Here's how the part is built. I have some questions about the finished solid (model axes, mm). Face numbers are marked on the shaded views. A direction names the side the tool comes from. Coordinates: 2 decimals unless noted, no trailing zeros. Loops run counter-clockwise (first coordinate to the right, second up) from the corner with the lowest first, then second, coordinate; pieces in that order, holes last. Notation, with made-up numbers: (-36, 28.5) - (-27, 28.5) arc R8 ccw to (-27, 34.5) - close; hole circle Ø2 at (26.5, 4.5). An arc over 180 degrees is marked (long way). Use a Markdown table: item, result.
```python
from build123d import *

# Parameters (mm, degrees)
BOSS_EXTRUDE1_DEPTH = 118.4275
SKETCH3_R           = 3.96875
SKETCH3_R_2         = 6.5
CUT_EXTRUDE1_DEPTH  = 25.4
SKETCH6_R           = 3.96875
CUT_EXTRUDE3_DEPTH  = 8.89
SKETCH4_R           = 4.7625
CUT_EXTRUDE2_DEPTH  = 6.35
SKETCH7_R           = 6.35
CUT_EXTRUDE4_DEPTH  = 2.54


with BuildPart() as part:
    # Sketch2 → Boss-Extrude1 (new body)
    with BuildSketch(Plane(origin=(0, 0, 0), x_dir=(0, 0, -1), z_dir=(1, 0, 0))):
        Polygon((0, -25.4), (0, 25.4), (-63.5, 25.4), (-63.5, 16.51), (-6.35, 16.51), (-6.35, -16.51), (-63.5, -16.51), (-63.5, -25.4), align=None)
    extrude(amount=BOSS_EXTRUDE1_DEPTH)

    # Sketch3 → Cut-Extrude1 (cut)
    with BuildSketch(Plane(origin=(0, 0, 0), x_dir=(1, 0, 0), z_dir=(0, 1, 0))):
        with Locations(Location((7.9375, -19.05, 0), (0, 0, 90))):
            Circle(SKETCH3_R)
        with Locations(Location((110.49, -19.05, 0), (0, 0, 90))):
            Circle(SKETCH3_R)
        with Locations(Location((38.1, -20.32, 0), (0, 0, 90))):
            Circle(SKETCH3_R_2)
        with BuildLine():
            Line((0, -63.5), (0, -19.05))
            ThreePointArc((0, -19.05), (1.173211717, -23.203108508), (4.346030936, -26.128506637))
            Line((4.346030936, -26.128506637), (30.73922523, -39.519797436))
            ThreePointArc((30.73922523, -39.519797436), (40.148824549, -41.564990827), (49.356556182, -38.747003333))
            Line((49.356556182, -38.747003333), (91.51717293, -12.752709815))
            ThreePointArc((91.51717293, -12.752709815), (93.758058641, -11.767067469), (96.182815356, -11.43))
            Line((96.182815356, -11.43), (98.7425, -11.43))
            ThreePointArc((98.7425, -11.43), (101.436576836, -12.545923164), (102.5525, -15.24))
            Line((102.5525, -15.24), (102.5525, -19.05))
            ThreePointArc((102.5525, -19.05), (110.49, -26.9875), (118.4275, -19.05))
            Line((118.4275, -19.05), (118.4275, -63.5))
            Line((118.4275, -63.5), (0, -63.5))
        make_face()
    extrude(amount=CUT_EXTRUDE1_DEPTH, mode=Mode.SUBTRACT)

    # Sketch6 → Cut-Extrude3 (cut)
    with BuildSketch(Plane.XZ.offset(25.4)):
        with Locations(Location((110.49, 19.05, 0), (0, 0, 270))):
            Circle(SKETCH6_R)
        with Locations(Location((7.9375, 19.05, 0), (0, 0, 270))):
            Circle(SKETCH6_R)
        with BuildLine():
            Line((0, 19.05), (0, 63.5))
            Line((0, 63.5), (118.4275, 63.5))
            Line((118.4275, 63.5), (118.4275, 19.05))
            ThreePointArc((118.4275, 19.05), (110.49, 26.9875), (102.5525, 19.05))
            Line((102.5525, 19.05), (102.5525, 15.24))
            ThreePointArc((102.5525, 15.24), (101.436576836, 12.545923164), (98.7425, 11.43))
            Line((98.7425, 11.43), (96.182815356, 11.43))
            ThreePointArc((96.182815356, 11.43), (93.758058641, 11.767067469), (91.51717293, 12.752709815))
            Line((91.51717293, 12.752709815), (60.419932998, 31.92583499))
            Line((60.419932998, 31.92583499), (15.772114941, 31.92583499))
            Line((15.772114941, 31.92583499), (4.346030936, 26.128506637))
            ThreePointArc((4.346030936, 26.128506637), (1.173211717, 23.203108508), (0, 19.05))
        make_face()
        with BuildLine():
            Line((25.6667, 27.370915615), (25.6667, 23.429084385))
            ThreePointArc((25.6667, 23.429084385), (20.0025, 25.4), (25.6667, 27.370915615))
        make_face()
    extrude(amount=-CUT_EXTRUDE3_DEPTH, mode=Mode.SUBTRACT)

    # Sketch4 → Cut-Extrude2 (cut)
    with BuildSketch(Plane.XY):
        with Locations(Location((19.05, 0, 0), (0, 0, 180))):
            Circle(SKETCH4_R)
        with Locations(Location((99.3775, 0, 0), (0, 0, 180))):
            Circle(SKETCH4_R)
    extrude(amount=CUT_EXTRUDE2_DEPTH, mode=Mode.SUBTRACT)

    # Sketch7 → Cut-Extrude4 (cut)
    with BuildSketch(Plane(origin=(0, -16.51, 0), x_dir=(1, 0, 0), z_dir=(0, 1, 0))):
        with Locations(Location((23.1775, -25.4, 0), (0, 0, 270))):
            Circle(SKETCH7_R)
    extrude(amount=-CUT_EXTRUDE4_DEPTH, mode=Mode.SUBTRACT)


solid = part.part
```
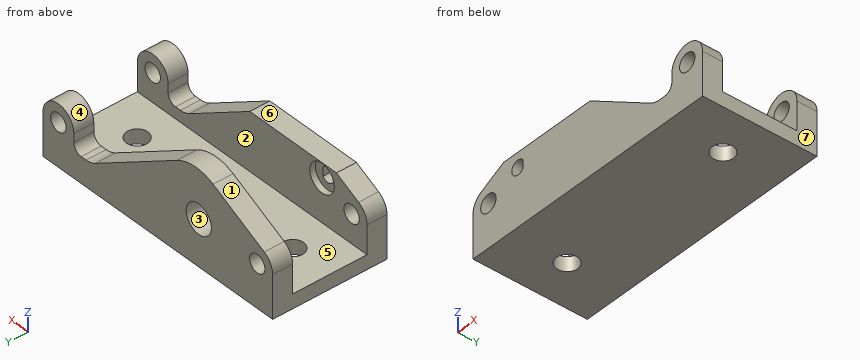
Q1. If we mould it in two halves opening along X, with no side actions, what happens to the marked faces 1, 2, 3 and 4? For each: pulls with the +X half, pulls with the -X half, needs draft (parallel to the pull), parting line crosses it, or undercut.
Check values:
| item | result |
|---|---|
| face 1 | pulls with the -X half |
| face 2 | needs draft |
| face 3 | undercut |
| face 4 | undercut |
Q2. Which directions (+Z, -Z, +X, -X, +Y, -Y) give clear straight access to the entire face, cutting with the end or side of a thin tool? Please do the marked faces 5, 6 and 7.
Check values:
| item | result |
|---|---|
| face 5 | +Z, +X, -X |
| face 6 | +Z, +X, -X, -Y |
| face 7 | +Z, -Z, +X, +Y, -Y |
Q3. I want a section at A-A, the plane y = 0. Give the number of separate pieces and of enclosed holes in the cut face, then the cut area to 3 significant figures.
Check values:
| item | result |
|---|---|
| separate pieces | 3 |
| enclosed holes | 0 |
| area | 631 mm^2 |
Q4. Will these pins go through, and if not, where does the flat tip stop? P1, Ø10, axis at x = 50, y = -17.5, coming from the +Z side; P2, Ø8, axis at x = 57.5, y = 2.5, coming from the +Z side; P3, Ø1.2, axis at y = -21.5, z = 26, coming from the -X side (3 decimals).
Check values:
| item | result |
|---|---|
| P1 | z = 31.93 |
| P2 | z = 6.35 |
| P3 | x = 3.175 |
Q5. I want a section at B-B, the plane x = 110.49. Write out the boundary of the cut face in (y, z), then the cut area to 3 significant figures.
Check values:
| item | result |
|---|---|
| outline | (-25.4, 0) - (25.4, 0) - (25.4, 15.08) - (16.51, 15.08) - (16.51, 6.35) - (-16.51, 6.35) - (-16.51, 15.08) - (-25.4, 15.08) - close; (-25.4, 23.02) - (-16.51, 23.02) - (-16.51, 26.99) - (-25.4, 26.99) - close; (16.51, 23.02) - (25.4, 23.02) - (25.4, 26.99) - (16.51, 26.99) - close |
| area | 548 mm^2 |
Q6. Please list where these lines run through material, in increasing order: L1, parallel to X at y = 23.75, z = 19.05; L2, parallel to Y at x = 67, z = 17; L3, parallel to Y at x = 24, z = 29. Write a range as from..to.
Check values:
| item | result |
|---|---|
| L1 | 0..3.97, 11.91..31.73, 44.47..81.3, 102.55..106.52, 114.46..118.43 |
| L2 | -25.4..-16.51, 16.51..25.4 |
| L3 | -25.4..-19.05, 16.51..25.4 |
